Here's how the part is built. I have some questions about the finished solid (model axes, mm). A direction names the side the tool comes from. Give positions to 0.01 mm unless a question says otherwise; leave off trailing zeros. Loops run counter-clockwise (first coordinate to the right, second up) from the corner with the lowest first, then second, coordinate; pieces in that order, holes last.
Q1. Suppose I cut it at A-A (z = 9.25). List the corners of the cut face in (x, y) for me, and give its area (3 significant figures).
Q2. Suppose I cut it at B-B (x = 0). List the corners of the cut face in (y, z) for me.
Q3. I'm going to push flat-ended pins straight in: P1, Ø8, axis at x = -12, y = 5, coming from the +Z side; P2, Ø3, axis at x = 8, y = 19.5, coming from the -Z side; P3, Ø0.5, axis at x = -19.5, z = 8.5, coming from the -Y side; P4, Ø4, axis at x = -9.5, z = 4, coming from the +Y side. Where does each tip first touch, or does it pass through?
Q4. I need wall thicknesses on probe 1 along X at (y, z) = (-0.5, 2.5); probe 2 along Z at (x, y) = (6.5, 12). Which ranges of each line are inside material? Lowest first, please.
Q5. For faces 1 (the face through (0, 0, 0)), 2 (the face through (0.326, 21.197, 8.465)), 3 (the face through (-20, -9.647, 8)), 4 (the face through (-0.362, -22.797, 8.465)), 5 (the face through (0.362, 22.797, 8.465)), which set-ups out of +Z, -Z, +X, -X, +Y, -Y let a thin tool reach every point of the face, with its end or its side?
Q6. Thinking about a two-plate mould opening in X: for faces 6 (the face through (20, 9.647, 8)), 7 (the face through (-5.344, -24.064, 2.958)), 8 (the face through (0, 0, 6)), which applies, pulls with the +X half, pulls with the -X half, needs draft (parallel to the pull), parting line crosses it, or undercut?
Q7. Suppose I cut it at C-C (y = 20.5). List the corners of the cut face in (x, z) for me.
Q8. Suppose I cut it at D-D (z = 1.5). List the corners of the cut face in (x, y) for me.
```python
from build123d import *

# Parameters (mm, degrees)
SKETCH1_R           = 24.65
BOSS_EXTRUDE1_DEPTH = 6
SKETCH2_R           = 22.8
SKETCH2_R_2         = 21.2
BOSS_EXTRUDE2_DEPTH = 5
CUT_EXTRUDE1_START  = -5
CUT_EXTRUDE1_DEPTH  = 5


with BuildPart() as part:
    # Sketch1 → Boss-Extrude1 (new body)
    with BuildSketch(Plane.XY):
        Circle(SKETCH1_R)
    extrude(amount=BOSS_EXTRUDE1_DEPTH)

    # Sketch2 → Boss-Extrude2 (add)
    with BuildSketch(Plane.XY.offset(6)):
        Circle(SKETCH2_R)
        Circle(SKETCH2_R_2, mode=Mode.SUBTRACT)
    extrude(amount=BOSS_EXTRUDE2_DEPTH)

    # Sketch3 → Cut-Extrude1 (cut)
    with BuildSketch(Plane.XY.offset(11).offset(CUT_EXTRUDE1_START)):
        with BuildLine():
            Line((-20.658461767, 9.647173545), (-18.877818798, 9.647173545))
            ThreePointArc((-18.877818798, 9.647173545), (-21.2, 0), (-18.877818798, -9.647173545))
            Line((-18.877818798, -9.647173545), (-20.658461767, -9.647173545))
            ThreePointArc((-20.658461767, -9.647173545), (-22.8, 0), (-20.658461767, 9.647173545))
        make_face()
        with BuildLine():
            Line((20.658461767, -9.647173545), (18.877818798, -9.647173545))
            ThreePointArc((18.877818798, -9.647173545), (21.2, 0), (18.877818798, 9.647173545))
            Line((18.877818798, 9.647173545), (20.658461767, 9.647173545))
            ThreePointArc((20.658461767, 9.647173545), (22.8, 0), (20.658461767, -9.647173545))
        make_face()
    extrude(amount=CUT_EXTRUDE1_DEPTH, mode=Mode.SUBTRACT)


solid = part.part
```
Solutions:
1. outline: (-20.66, -9.65) arc R22.8 ccw to (20.66, -9.65) - (18.88, -9.65) arc R21.2 cw to (-18.88, -9.65) - close; (-20.66, 9.65) - (-18.88, 9.65) arc R21.2 cw to (18.88, 9.65) - (20.66, 9.65) arc R22.8 ccw to start
1. area: 157 mm2
2. outline: (-24.65, 0) - (24.65, 0) - (24.65, 6) - (22.8, 6) - (22.8, 11) - (21.2, 11) - (21.2, 6) - (-21.2, 6) - (-21.2, 11) - (-22.8, 11) - (-22.8, 6) - (-24.65, 6) - close
3. P1: stops at z = 6
3. P2: stops at z = 0
3. P3: stops at y = -12.22
3. P4: stops at y = 23.48
4. probe 1: x = -24.64 to 24.64
4. probe 2: z = 0 to 6
5. face 1: -Z, +X, -X, +Y, -Y
5. face 2: +Z
5. face 3: +Z, +X, -X
5. face 4: +Z, -Y
5. face 5: +Z, +Y
6. face 6: needs draft
6. face 7: parting line crosses it
6. face 8: undercut
7. outline: (-13.69, 0) - (13.69, 0) - (13.69, 6) - (9.98, 6) - (9.98, 11) - (5.4, 11) - (5.4, 6) - (-5.4, 6) - (-5.4, 11) - (-9.98, 11) - (-9.98, 6) - (-13.69, 6) - close
8. outline: circle Ø49.3 at (0, 0)
